Read the model definition and answer for the solid it produces. Units are mm, in the model's axes. A direction names the side the tool comes from. Coordinates: 2 decimals unless noted, no trailing zeros. Order: outer loops, then holes, each group sorted by start corner. A loop starts at its lowest first (then second) coordinate and runs counter-clockwise, first axis right, second up. Notation, with made-up numbers: M 37,23.5 L 52,23.5 A12 ccw 52,46.5 Z; hole C 51.25,50 d6. An arc over 180 degrees is marked long. Write each question's results on one line, items separated by ' | '.
```python
from build123d import *

# Parameters (mm, degrees)
BOSS_EXTRUDE1_DEPTH      = 2.4
BOSS_EXTRUDE2_DEPTH      = 2.2
BOSS_EXTRUDE2_DEPTH_BACK = 2.2
SKETCH3_R                = 1.125
CUT_EXTRUDE1_DEPTH       = 27.620762574
SKETCH4_W                = 5.3
SKETCH4_H                = 1.3
CUT_EXTRUDE2_DEPTH       = 38.364588851
FILLET1_R                = 1.6
FILLET2_R                = 0.25
FILLET3_R                = 1
SKETCH5_R                = 1.75
CUT_EXTRUDE3_DEPTH       = 27.620762574


with BuildPart() as part:
    # Sketch1 → Boss-Extrude1 (new body)
    with BuildSketch(Plane(origin=(0, 0, 0), x_dir=(1, 0, 0), z_dir=(0, 1, 0))):
        with BuildLine():
            Line((-8.75, 16), (-8.75, 19.25))
            Line((-8.75, 19.25), (8.75, 19.25))
            Line((8.75, 19.25), (8.75, 16))
            ThreePointArc((8.75, 16), (9.701902961, 13.701902961), (12, 12.75))
            Line((12, 12.75), (15.25, 12.75))
            Line((15.25, 12.75), (15.25, -4.6))
            Line((15.25, -4.6), (12, -4.6))
            ThreePointArc((12, -4.6), (8.75, -7.85), (12, -11.1))
            Line((12, -11.1), (15.25, -11.1))
            Line((15.25, -11.1), (15.25, -19.25))
            Line((15.25, -19.25), (-15.25, -19.25))
            Line((-15.25, -19.25), (-15.25, -11.1))
            Line((-15.25, -11.1), (-12, -11.1))
            ThreePointArc((-12, -11.1), (-8.75, -7.85), (-12, -4.6))
            Line((-12, -4.6), (-15.25, -4.6))
            Line((-15.25, -4.6), (-15.25, 12.75))
            Line((-15.25, 12.75), (-12, 12.75))
            ThreePointArc((-12, 12.75), (-9.701902961, 13.701902961), (-8.75, 16))
        make_face()
    extrude(amount=BOSS_EXTRUDE1_DEPTH)

    # Sketch2 → Boss-Extrude2 (add, two sides: drawn at the far end of the back side and taken through both)
    with BuildSketch(Plane(origin=(0, 0, -19.25), x_dir=(-1, 0, 0), z_dir=(0, 0, -1)).offset(-BOSS_EXTRUDE2_DEPTH_BACK)):
        Polygon((0, 0), (5.75, 0), (5.75, -1.6), (-5.75, -1.6), (-5.75, 0), align=None)
    extrude(amount=BOSS_EXTRUDE2_DEPTH + BOSS_EXTRUDE2_DEPTH_BACK)

    # Sketch3 → Cut-Extrude1 (cut, through all)
    with BuildSketch(Plane(origin=(0, 2.4, 0), x_dir=(1, 0, 0), z_dir=(0, 1, 0))):
        with Locations(Location((-12, -16.25, 0), (0, 0, 270))):
            Circle(SKETCH3_R)
        with Locations(Location((12, -16.25, 0), (0, 0, 270))):
            Circle(SKETCH3_R)
    extrude(amount=-CUT_EXTRUDE1_DEPTH, mode=Mode.SUBTRACT)

    # Sketch4 → Cut-Extrude2 (cut, through all)
    with BuildSketch(Plane.ZY.offset(15.25)):
        with Locations((16.6, 1.75)):
            Rectangle(SKETCH4_W, SKETCH4_H)
    extrude(amount=-CUT_EXTRUDE2_DEPTH, mode=Mode.SUBTRACT)

    # Fillet1
    fillet1_edges = [part.edges().sort_by_distance(p)[0] for p in [
        (15.25, 0.55, 19.25),
        (-15.25, 0.55, 19.25),
    ]]
    fillet(fillet1_edges, radius=FILLET1_R)

    # Fillet2
    fillet2_edges = [part.edges().sort_by_distance(p)[0] for p in [
        (0, 0, -19.25),
    ]]
    fillet(fillet2_edges, radius=FILLET2_R)

    # Fillet3
    fillet3_edges = [part.edges().sort_by_distance(p)[0] for p in [
        (0, 0, -17.05),
    ]]
    fillet(fillet3_edges, radius=FILLET3_R)

    # Sketch5 → Cut-Extrude3 (cut, through all)
    with BuildSketch(Plane(origin=(0, 2.4, 0), x_dir=(1, 0, 0), z_dir=(0, 1, 0))):
        with Locations(Location((-6.475522352, 6.733497746, 0), (0, 0, 270))):
            Circle(SKETCH5_R)
        with Locations(Location((-10.634056634, 6.888687884, 0), (0, 0, 270))):
            Circle(SKETCH5_R)
        with Locations(Location((-7.802519248, 11.828753503, 0), (0, 0, 270))):
            Circle(SKETCH5_R)
        with Locations(Location((-6.458727551, 1.375956017, 0), (0, 0, 270))):
            Circle(SKETCH5_R)
        with Locations(Location((-2.658497746, -2.400522352, 0), (0, 0, 270))):
            Circle(SKETCH5_R)
        with Locations(Location((2.699043983, -2.383727551, 0), (0, 0, 270))):
            Circle(SKETCH5_R)
        with Locations(Location((6.475522352, 1.416502254, 0), (0, 0, 270))):
            Circle(SKETCH5_R)
        with Locations(Location((6.458727551, 6.774043983, 0), (0, 0, 270))):
            Circle(SKETCH5_R)
        with Locations(Location((2.658497746, 10.550522352, 0), (0, 0, 270))):
            Circle(SKETCH5_R)
        with Locations(Location((-2.699043983, 10.533727551, 0), (0, 0, 270))):
            Circle(SKETCH5_R)
        with Locations(Location((-2.880303131, 14.691207132, 0), (0, 0, 270))):
            Circle(SKETCH5_R)
        with Locations(Location((2.813687884, 14.709056634, 0), (0, 0, 270))):
            Circle(SKETCH5_R)
        with Locations(Location((7.753753503, 11.877519248, 0), (0, 0, 270))):
            Circle(SKETCH5_R)
        with Locations(Location((10.616207132, 6.955303131, 0), (0, 0, 270))):
            Circle(SKETCH5_R)
        with Locations(Location((10.634056634, 1.261312116, 0), (0, 0, 270))):
            Circle(SKETCH5_R)
        with Locations(Location((7.802519248, -3.678753503, 0), (0, 0, 270))):
            Circle(SKETCH5_R)
        with Locations(Location((2.880303131, -6.541207132, 0), (0, 0, 270))):
            Circle(SKETCH5_R)
        with Locations(Location((-2.813687884, -6.559056634, 0), (0, 0, 270))):
            Circle(SKETCH5_R)
        with Locations(Location((-7.753753503, -3.727519248, 0), (0, 0, 270))):
            Circle(SKETCH5_R)
        with Locations(Location((-10.616207132, 1.194696869, 0), (0, 0, 270))):
            Circle(SKETCH5_R)
    extrude(amount=-CUT_EXTRUDE3_DEPTH, mode=Mode.SUBTRACT)


solid = part.part
```
(1) Straight lines are drawn through the part: line 1 (Z direction, x = 14, y = 1.3); line 2 (X direction, y = 1.8, z = -5.5); line 3 (X direction, y = 1.7, z = -8). For each, find the intervals that lie inside material, in ascending order.
Conclusion:
line 1: -12.75 to 4.6, 11.1 to 13.95 | line 2: -15.25 to -11.7, -9.57 to -7.72, -5.23 to 5.26, 7.66 to 9.64, 11.59 to 15.25 | line 3: -15.25 to -11.99, -9.28 to -7.68, -5.27 to 5.21, 7.71 to 9.21, 12.02 to 15.25
(2) The part is cut by section C-C, the plane z = -11. Write down the section's boundary in (x, y), then the cut area to 3 significant figures.
Conclusion:
outline: M -15.25,0 L -9.34,0 L -9.34,2.4 L -15.25,2.4 Z; M -6.26,0 L -4.39,0 L -4.39,2.4 L -6.26,2.4 Z; M -1.01,0 L 0.97,0 L 0.97,2.4 L -1.01,2.4 Z; M 4.35,0 L 6.24,0 L 6.24,2.4 L 4.35,2.4 Z; M 9.27,0 L 15.25,0 L 15.25,2.4 L 9.27,2.4 Z | area: 42.3 mm²
(3) The part is cut by section A-A, the plane z = 16.25. Write down the section's boundary in (x, y) (3 decimals), then the cut area to 3 significant figures.
Conclusion:
outline: M -15.25,0 L -13.125,0 L -13.125,1.1 L -15.25,1.1 Z; M -10.875,0 L 10.875,0 L 10.875,1.1 L -10.875,1.1 Z; M 13.125,0 L 15.25,0 L 15.25,1.1 L 13.125,1.1 Z | area: 28.6 mm²
(4) The part is cut by section D-D, the plane z = -2.5. Write down the section's boundary in (x, y).
Conclusion:
outline: M -15.25,0 L -11.78,0 L -11.78,2.4 L -15.25,2.4 Z; M -9.45,0 L -7.8,0 L -7.8,2.4 L -9.45,2.4 Z; M -5.12,0 L 5.1,0 L 5.1,2.4 L -5.12,2.4 Z; M 7.85,0 L 9.4,0 L 9.4,2.4 L 7.85,2.4 Z; M 11.87,0 L 15.25,0 L 15.25,2.4 L 11.87,2.4 Z
(5) The mould has two halves that part along Z. Classify faces 1 (the flat face through (-15.25, 0.9, 13.7)), 2 (the cylindrical face through (-6.6, 1.2, -13.1)), 3 (the flat face through (14, 1, -12.75)): pulls with the +Z half, pulls with the -Z half, needs draft (parallel to the pull), parting line crosses it, or undercut.
Conclusion:
face 1: needs draft | face 2: undercut | face 3: pulls with the -Z half
(6) For faces 4 (the flat face through (14, 1, 4.6)), 5 (the cylindrical face through (7.083, 1.217, -10.261)), 6 (the flat face through (0, 2, 13.95)), determine the directions among +Z, -Z, +X, -X, +Y, -Y from which every point of the face is accessible in a straight line to the end or side of a thin tool.
Conclusion:
face 4: +X, +Y, -Y | face 5: +Y, -Y | face 6: +Z, +X, -X, +Y
(7) Given pin 1 (4 mm diameter, centred on x = -8, z = 6.5, fed in from -Y); pin 2 (3 mm diameter, centred on x = -2.81, z = 6.56, fed in from +Y); pin 3 (0.7 mm diameter, centred on x = -13.5, y = 1, fed in from -Z), each flat-ended and moving along its own axis, determine where each tip first touches the part or whether it passes through.
Conclusion:
pin 1: y = 0 | pin 2: through | pin 3: z = -12.75
(8) The part is cut by section B-B, the plane x = -10. Write down the section's boundary in (y, z), then the cut area to 3 significant figures.
Conclusion:
outline: M 0,-13.44 L 2.4,-13.44 L 2.4,-8.52 L 0,-8.52 Z; M 0,-5.26 L 2.4,-5.26 L 2.4,-2.83 L 0,-2.83 Z; M 0,0.44 L 2.4,0.44 L 2.4,5.29 L 0,5.29 Z; M 0,10.41 L 2.4,10.41 L 2.4,13.95 L 1.1,13.95 L 1.1,19.25 L 0,19.25 Z | area: 43.6 mm²
